Autodesk Inventor part; units mm, degrees
ref_plane "YZ Plane" through (0, 0, 0) normal (1, 0, 0) x (0, 1, 0)
ref_plane "XZ Plane" through (0, 0, 0) normal (0, 1, 0) x (-1, 0, 0)
ref_plane "XY Plane" through (0, 0, 0) normal (0, 0, 1) x (1, 0, 0)
sketch "Sketch1" plane through (0, 0, 0) normal (1, 0, 0) x (0, 1, 0)
  line L0 (0, 0) -> (5, 0)
  line L1 (5, 0) -> (5, -10)
  line L2 (5, -10) -> (2.5, -7.5)
  line L3 (2.5, -7.5) -> (0, -10)
  line L4 (0, 0) -> (0, -10)
  line L5 (2.5, -7.5) -> (2.5, -12.5) construction
  circle A0 centre (2.5, -10.3284) radius 2 construction
  line L6 (2.5, -10.3284) -> (1.25, -10.3284) construction
  line L7 (5, -10.6569) -> (2.5, -13.1569) construction
  line L8 (2.5, -13.1569) -> (0, -10.6569) construction
  dimension "d0" = 5
  dimension "d3" = 10
  dimension "d4" = 4
  dimension "d33" = 0.6569
  dimension "d34" = 5.6569
  dimension "d35" = 2.8284
extrude "Extrusion1" add sketch "Sketch1" along normal blind 100
sketch "Sketch2" plane through (0, 5, 0) normal (0, 1, 0) x (1, 0, 0)
  line L0 (0, 10) -> (0, 0) construction
  line L1 (0, 0) -> (100, 0) construction
  line L2 (0, 10) -> (100, 10) construction
  line L3 (4, 0) -> (4, 10) construction
  line L4 (50, 0) -> (50, 15) construction
  circle A0 centre (4, 4) radius 2
  circle A1 centre (96, 4) radius 2
  point P0 (0, 5)
  dimension "d8" = 10
  dimension "d10" = 4
  dimension "d12" = 15
  dimension "d13" = 50
  dimension "d14" = 4
  dimension "d15" = 4
hole "Hole1" at (4, 5, -4) direction (0, -1, 0) diameter 3.4587 end through all
hole "Hole2" at (96, 5, -4) direction (0, -1, 0) diameter 3.4587 end through all
chamfer "Chamfer2" distance 0.4 angle 45 2 edges at (4, 5, -5.7294) (96, 5, -5.7294)
sketch "Sketch3" plane through (0, 0, 0) normal (0, 0, 1) x (1, 0, 0)
  line L0 (0, 5) -> (100, 5)
  line L1 (0, 0) -> (100, 0)
  line L2 (8, 5) -> (92, 5)
  line L3 (92, 5) -> (92, 0)
  line L4 (92, 0) -> (8, 0)
  line L5 (8, 0) -> (8, 5)
  line L6 (0, 5) -> (0, 0)
  point P0 (0, 2.5)
  point P1 (8, 0)
  point P2 (92, 5)
  dimension "d39" = 84
  dimension "d40" = 8
extrude "Extrusion2" cut sketch "Sketch3" against normal blind 6 contours L0 L3 L1 L5
properties part number "K-tor-kulek-blatu" material "Steel, High Strength, Low Alloy"
Build history of the part. All positions in model axes, mm. A direction names the side the tool comes from. Give positions to 0.01 mm unless a question says otherwise; leave off trailing zeros. Order: outer loops, then holes, each group sorted by start corner. A loop starts at its lowest first (then second) coordinate and runs counter-clockwise, first axis right, second up. Notation, with made-up numbers: M -24.5,-27 L -15.5,-27 A22 cw -15.5,-16 Z; hole C 87.5,-1.75 d10. An arc over 180 degrees is marked long. Write item = value, one per line. Start each with the question number.
(1) Slice it at B-B on x = 96. Write the cut outline in (y, z).
(2) Slice it at C-C on y = 1.2. Write the cut outline in (x, z), plus the area to 3 significant figures.
(3) Which spindle directions (+Z, -Z, +X, -X, +Y, -Y) get a long thin tool onto all of the face, cutting with end or side? Do faces 5 (the flat face through (49, 3, -6)), 6 (the cylindrical face through (94.285, 2.268, -4.225)), 7 (the flat face through (49, 4, -9)). Say none if no direction does.
(4) Two-plate mould, pull along X, no slides. Class faces 1 (the flat face through (100, 2, -4)), 2 (the flat face through (92, 3, -3)), 3 (the flat face through (49, 0, -7)), 4 (the flat face through (0, 2, -4)): released by +X, released by -X, zero draft, split by the parting line, or undercut.
(5) Pin check, flat tip, straight feed: pin 1 Ø3 at (x, z) = (96, -4) entering from -Y. Stop position of the tip, or through.
(6) Probe L1, parallel to X at y = 1.4, z = -4; L2, parallel to X at y = 1.4, z = -4.75; L3, parallel to X at y = 0.65, z = -2. List the from-to ranges inside material, lowest first. Write a range as [from, to].
(7) Slice it at D-D on x = 26.5. Write the cut outline in (y, z).
(8) Slice it at A-A on z = -4. Write the cut outline in (x, y), plus the area to 3 significant figures.
Responses:
q1.outline = M 0,-10 L 2.5,-7.5 L 5,-10 L 5,-6.13 L 4.6,-5.73 L 0,-5.73 Z; M 0,-2.27 L 4.6,-2.27 L 5,-1.87 L 5,0 L 0,0 Z
q2.outline = M 0,-8.8 L 100,-8.8 L 100,0 L 92,0 L 92,-6 L 8,-6 L 8,0 L 0,0 Z; hole C 4,-4 d3.46; hole C 96,-4 d3.46
q2.area = 357 mm2
q3.face_5 = +Z, +Y, -Y
q3.face_6 = +Y, -Y
q3.face_7 = -Z, +X, -X
q4.face_1 = released by +X
q4.face_2 = undercut
q4.face_3 = zero draft
q4.face_4 = released by -X
q5.pin_1 = through
q6.L1 = [0, 2.27], [5.73, 8], [92, 94.27], [97.73, 100]
q6.L2 = [0, 2.44], [5.56, 8], [92, 94.44], [97.56, 100]
q6.L3 = [0, 8], [92, 100]
q7.outline = M 0,-10 L 2.5,-7.5 L 5,-10 L 5,-6 L 0,-6 Z
q8.outline = M 0,0 L 2.27,0 L 2.27,4.6 L 1.87,5 L 0,5 Z; M 5.73,0 L 8,0 L 8,5 L 6.13,5 L 5.73,4.6 Z; M 92,0 L 94.27,0 L 94.27,4.6 L 93.87,5 L 92,5 Z; M 97.73,0 L 100,0 L 100,5 L 98.13,5 L 97.73,4.6 Z
q8.area = 45.1 mm2
